from build123d import *

# Parameters (mm, degrees)
CROQUIS1_W              = 94
CROQUIS1_H              = 84
CROQUIS1_R              = 7.445624545
SALIENTE_EXTRUIR1_DEPTH = 2.5
REDONDEO1_R             = 6


with BuildPart() as part:
    # Croquis1 → Saliente-Extruir1 (new body)
    with BuildSketch(Plane.XY):
        with Locations((-17.9, 28.75)):
            Rectangle(CROQUIS1_W, CROQUIS1_H)
        with Locations((6.65, 28.75)):
            Circle(CROQUIS1_R, mode=Mode.SUBTRACT)
    extrude(amount=SALIENTE_EXTRUIR1_DEPTH)

    # Redondeo1
    redondeo1_edges = [part.edges().sort_by_distance(p)[0] for p in [
        (-64.9, 70.75, 1.25),
        (29.1, 70.75, 1.25),
        (29.1, -13.25, 1.25),
        (-64.9, -13.25, 1.25),
    ]]
    fillet(redondeo1_edges, radius=REDONDEO1_R)


solid = part.part
Verification items for the finished model (mm, model axes). Give positions to 0.01 mm unless a question says otherwise; leave off trailing zeros. Loops run counter-clockwise (first coordinate to the right, second up) from the corner with the lowest first, then second, coordinate; pieces in that order, holes last. Notation, with made-up numbers: (21, -14) - (73, -14) arc R22 cw to (73, -2) - close; hole circle Ø9 at (61, -35.5). An arc over 180 degrees is marked (long way). Write item = value, one per line. Start each with the question number.
Q1. Thickness scan on line 1 (Y direction, x = 6.65, z = 1); line 2 (Y direction, x = 1.5, z = 0.6); line 3 (X direction, y = 24, z = 1.4). Record the ranges inside material, lowest first.
Q2. Cross-section at B-B, the plane y = 28.75. Enter the section's corners in (x, z), and give its area (3 significant figures).
Q3. Cross-section at C-C, the plane x = 6.65. Enter the section's corners in (y, z), and give its area (3 significant figures).
Q4. Cross-section at A-A, the plane z = 0.4. Enter the section's corners in (x, y), and give its area (3 significant figures).
Answer key:
q1.line_1 = -13.25 to 21.3, 36.2 to 70.75
q1.line_2 = -13.25 to 23.37, 34.13 to 70.75
q1.line_3 = -64.9 to 0.92, 12.38 to 29.1
q2.outline = (-64.9, 0) - (-0.8, 0) - (-0.8, 2.5) - (-64.9, 2.5) - close; (14.1, 0) - (29.1, 0) - (29.1, 2.5) - (14.1, 2.5) - close
q2.area = 198 mm^2
q3.outline = (-13.25, 0) - (21.3, 0) - (21.3, 2.5) - (-13.25, 2.5) - close; (36.2, 0) - (70.75, 0) - (70.75, 2.5) - (36.2, 2.5) - close
q3.area = 173 mm^2
q4.outline = (-64.9, -7.25) arc R6 ccw to (-58.9, -13.25) - (23.1, -13.25) arc R6 ccw to (29.1, -7.25) - (29.1, 64.75) arc R6 ccw to (23.1, 70.75) - (-58.9, 70.75) arc R6 ccw to (-64.9, 64.75) - close; hole circle Ø14.89 at (6.65, 28.75)
q4.area = 7,690 mm^2
